from build123d import *

# Parameters (mm, degrees)
F0_W     = 12.7
F0_H     = 151.13
F1_DEPTH = 3.175
F0_H_2   = 3.175
F2_DEPTH = 93.98
F0_H_3   = 12.7
F0_R     = 1.905
F3_DEPTH = 3.175
F4_W     = 12.7
F4_H     = 3.175
F5_DEPTH = 9.525
F6_W     = 12.7
F6_H     = 3.175
F7_DEPTH = 9.525
F9_DEPTH = 1.55575


with BuildPart() as f1:
    # F0 (on Top) → F1 (new body)
    with BuildSketch(Plane.XY):
        Rectangle(F0_W, F0_H)
    extrude(amount=F1_DEPTH)

    # F0 (on Top) → F2 (join)
    with BuildSketch(Plane.XY):
        with Locations((0, 77.1525)):
            Rectangle(F0_W, F0_H_2)
        with Locations((0, -77.1525)):
            Rectangle(F0_W, F0_H_2)
    extrude(amount=F2_DEPTH)

    # F0 (on Top) → F3 (join)
    with BuildSketch(Plane.XY):
        with Locations((0, 85.09)):
            Rectangle(F0_W, F0_H_3)
        with Locations((0, 85.09)):
            Circle(F0_R, mode=Mode.SUBTRACT)
        with Locations((0, -85.09)):
            Rectangle(F0_W, F0_H_3)
        with Locations((0, -85.09)):
            Circle(F0_R, mode=Mode.SUBTRACT)
    extrude(amount=F3_DEPTH)

    # F4 (on face) → F5 (join)
    with BuildSketch(Plane.XZ.offset(-75.565)):
        with Locations((0, 92.3925)):
            Rectangle(F4_W, F4_H)
    extrude(amount=F5_DEPTH)

    # F6 (on face) → F7 (join)
    with BuildSketch(Plane(origin=(0, -75.565, 0), x_dir=(-1, 0, 0), z_dir=(0, 1, 0))):
        with Locations((0, 92.3925)):
            Rectangle(F6_W, F6_H)
    extrude(amount=F7_DEPTH)

    # F8 (on face) → F9 (join)
    with BuildSketch(Plane.YZ.offset(6.35)):
        Polygon((75.565, 28.575), (50.165, 3.175), (75.565, 3.175), align=None)
        Polygon((-75.565, 3.175), (-50.165, 3.175), (-75.565, 28.575), align=None)
    extrude(amount=-F9_DEPTH)


solid = f1.part
Model file for the job. Use its own axes, mm. A direction names the side the tool comes from. Round coordinates to 2 decimals unless told otherwise and drop trailing zeros. Loops run counter-clockwise (first coordinate to the right, second up) from the corner with the lowest first, then second, coordinate; pieces in that order, holes last. Notation, with made-up numbers: M 4,-10.5 L 46,-10.5 A22 cw 46,12.5 Z; hole C -34,56.5 d8. An arc over 180 degrees is marked long. One line per question, with ' | ' between items.
1) Flat gauge pins, fed straight in: pin 1 (1.6 mm diameter, centred on x = -1.5, z = 93, fed in from -Y); pin 2 (4 mm diameter, centred on x = -3, z = 36.5, fed in from +Y); pin 3 (1.5 mm diameter, centred on x = -3.5, y = 46, fed in from +Z) (3 decimals). Where does each tip first touch, or does it go through?
Solved:
pin 1: stops at y = -78.74 | pin 2: stops at y = 78.74 | pin 3: stops at z = 3.175
2) 3-axis set-ups, long thin cutter, end or side, ignore diameter. For faces 4 (the flat face through (5.58, 63.04, 16.05)), 5 (the flat face through (0, 78.74, 48)), 6 (the flat face through (0, -78.74, 48)), 7 (the flat face through (4.794, 68, 10)), 8 (the flat face through (-6.35, 0, 2)): which of +Z, -Z, +X, -X, +Y, -Y reach the whole face in a straight line?
Solved:
face 4: +X, -X | face 5: +Z, +X, -X, +Y | face 6: +Z, +X, -X, -Y | face 7: -X | face 8: +Z, -Z, -X, +Y, -Y
3) Band-saw the part on B-B (x = 0). Give the cut face in (y, z) (3 decimals), then the cut area to 3 significant figures.
Solved:
outline: M -91.44,0 L -86.995,0 L -86.995,3.175 L -91.44,3.175 Z; M -83.185,0 L 83.185,0 L 83.185,3.175 L 78.74,3.175 L 78.74,93.98 L 66.04,93.98 L 66.04,90.805 L 75.565,90.805 L 75.565,3.175 L -75.565,3.175 L -75.565,90.805 L -66.04,90.805 L -66.04,93.98 L -78.74,93.98 L -78.74,3.175 L -83.185,3.175 Z; M 86.995,0 L 91.44,0 L 91.44,3.175 L 86.995,3.175 Z | area: 1,190 mm²
4) Drill centre lines: line 1 along Y through (x, z) = (0, 0.85) (3 decimals); line 2 along Y through (x, z) = (1, 40) (3 decimals); line 3 along Z through (x, y) = (-4.75, -70) (3 decimals). Where is each one in solid material? Low to high.
Solved:
line 1: y = -91.44 to -86.995, -83.185 to 83.185, 86.995 to 91.44 | line 2: y = -78.74 to -75.565, 75.565 to 78.74 | line 3: z = 0 to 3.175, 90.805 to 93.98
5) Band-saw the part on A-A (z = 53). Give the cut face in (x, y) (3 decimals), then the cut area to 3 significant figures.
Solved:
outline: M -6.35,-78.74 L 6.35,-78.74 L 6.35,-75.565 L -6.35,-75.565 Z; M -6.35,75.565 L 6.35,75.565 L 6.35,78.74 L -6.35,78.74 Z | area: 80.6 mm²
6) Band-saw the part on D-D (z = 19). Give the cut face in (x, y) (3 decimals), then the cut area to 3 significant figures.
Solved:
outline: M -6.35,-78.74 L 6.35,-78.74 L 6.35,-65.99 L 4.794,-65.99 L 4.794,-75.565 L -6.35,-75.565 Z; M -6.35,75.565 L 4.794,75.565 L 4.794,65.99 L 6.35,65.99 L 6.35,78.74 L -6.35,78.74 Z | area: 110 mm²
7) Band-saw the part on C-C (y = -85.09). Give the cut face in (x, z) (3 decimals), then the cut area to 3 significant figures.
Solved:
outline: M -6.35,0 L -1.905,0 L -1.905,3.175 L -6.35,3.175 Z; M 1.905,0 L 6.35,0 L 6.35,3.175 L 1.905,3.175 Z | area: 28.2 mm²
8) Mould opens along Y. For faces 1 (the flat face through (-2, 87, 3.175)), 2 (the flat face through (0, 1, 3.175)), 3 (the flat face through (0, 91.44, 2)) say: +Y half, -Y half, draft (parallel to the pull), parting line (faces both ways), or undercut.
Solved:
face 1: draft | face 2: undercut | face 3: +Y half
